Could you check a few things on this model? Use its own coordinates, in mm. A direction names the side the tool comes from. Round coordinates to 2 decimals unless told otherwise and drop trailing zeros. Write each loop counter-clockwise with the first axis right and the second up, starting at its lowest first coordinate (ties: lowest second). Pieces come first, ordered by that corner, then holes. Notation, with made-up numbers: M 8.5,1.5 L 12.5,1.5 A29 ccw 12.5,40.5 Z; hole C 17.25,19.25 d4. An arc over 180 degrees is marked long. One line per item, written item: value. Start each with the question number.
(1) I want a section at D-D on x = 17. Please give me the cut outline in (y, z).
(2) If I drill on L1, parallel to X at y = 7.5, z = 15; L2, parallel to X at y = 1.6, z = 0; L3, parallel to Z at x = 0, y = 6.5, over which ranges is the centre line in solid material (lowest first)?
(3) Which directions (+Z, -Z, +X, -X, +Y, -Y) give clear straight access to the entire face, cutting with the end or side of a thin tool? Please do faces 4 (the face through (4, 3, 1)), 5 (the face through (0, 5, -20)), 6 (the face through (0, 8, -12)).
(4) I want a section at A-A on x = 5. Please give me the cut outline in (y, z), and give its area (3 significant figures).
(5) I want a section at B-B on z = 15. Please give me the cut outline in (x, y), and give its area (3 significant figures).
(6) Thinking about a two-plate mould opening in Z: for faces 1 (the face through (-4, 2, 0)), 2 (the face through (0, 5, 20)), 3 (the face through (0, 11, 17)), which applies, released by +Z, released by -Z, zero draft, split by the parting line, or undercut?
(7) I want a section at C-C on y = 8.5. Please give me the cut outline in (x, z), and give its area (3 significant figures).
(8) I'm going to push flat-ended pins straight in: pin 1 Ø1.2 at (x, z) = (-5, 0.5) entering from +Y; pin 2 Ø12 at (x, z) = (10.5, -2.5) entering from +Y; pin 3 Ø1.8 at (x, z) = (17, -15) entering from +Y. Where does each tip first touch, or does it pass through?
```python
from build123d import *

# Parameters (mm, degrees)
SKETCH1_W               = 50
SKETCH1_H               = 40
BOSS_EXTRUDE1_DEPTH     = 5
SKETCH2_R               = 1
CUT_EXTRUDE1_DEPTH      = 33.403703492
SKETCH3_R               = 2
CUT_EXTRUDE2_DEPTH      = 2
SKETCH5_W               = 50
SKETCH5_H               = 8
BOSS_EXTRUDE2_DEPTH     = 6
CUT_EXTRUDE3_DEPTH      = 33.57299495
CUT_EXTRUDE3_DEPTH_BACK = 33.57299495
SKETCH4_R               = 1


with BuildPart() as part:
    # Sketch1 → Boss-Extrude1 (new body)
    with BuildSketch(Plane(origin=(0, 0, 0), x_dir=(1, 0, 0), z_dir=(0, 1, 0))):
        Rectangle(SKETCH1_W, SKETCH1_H)
    extrude(amount=BOSS_EXTRUDE1_DEPTH)

    # Sketch2 → Cut-Extrude1 (cut, through all)
    with BuildSketch(Plane(origin=(0, 5, 0), x_dir=(1, 0, 0), z_dir=(0, 1, 0))):
        with Locations(Location((-5, 0, 0), (0, 0, 270))):
            Circle(SKETCH2_R)
        with Locations(Location((5, 0, 0), (0, 0, 270))):
            Circle(SKETCH2_R)
    extrude(amount=-CUT_EXTRUDE1_DEPTH, mode=Mode.SUBTRACT)

    # Sketch3 → Cut-Extrude2 (cut)
    with BuildSketch(Plane(origin=(0, 5, 0), x_dir=(1, 0, 0), z_dir=(0, 1, 0))):
        with Locations(Location((-5, 0, 0), (0, 0, 270))):
            Circle(SKETCH3_R)
        with Locations(Location((5, 0, 0), (0, 0, 270))):
            Circle(SKETCH3_R)
    extrude(amount=-CUT_EXTRUDE2_DEPTH, mode=Mode.SUBTRACT)

    # Sketch5 → Boss-Extrude2 (add)
    with BuildSketch(Plane(origin=(0, 5, 0), x_dir=(1, 0, 0), z_dir=(0, 1, 0))):
        with Locations((0, 16)):
            Rectangle(SKETCH5_W, SKETCH5_H)
        with Locations((0, -16)):
            Rectangle(SKETCH5_W, SKETCH5_H)
    extrude(amount=BOSS_EXTRUDE2_DEPTH)

    # Sketch4 → Cut-Extrude3 (cut, two sides: drawn at the far end of the back side and taken through both)
    with BuildSketch(Plane(origin=(0, 5, 0), x_dir=(1, 0, 0), z_dir=(0, 1, 0)).offset(-CUT_EXTRUDE3_DEPTH_BACK)):
        with Locations(Location((-17, 15, 0), (0, 0, 270))):
            Circle(SKETCH4_R)
        with Locations(Location((0, 15, 0), (0, 0, 270))):
            Circle(SKETCH4_R)
        with Locations(Location((17, 15, 0), (0, 0, 270))):
            Circle(SKETCH4_R)
        with Locations(Location((-17, -15, 0), (0, 0, 270))):
            Circle(SKETCH4_R)
        with Locations(Location((0, -15, 0), (0, 0, 270))):
            Circle(SKETCH4_R)
        with Locations(Location((17, -15, 0), (0, 0, 270))):
            Circle(SKETCH4_R)
    extrude(amount=CUT_EXTRUDE3_DEPTH + CUT_EXTRUDE3_DEPTH_BACK, mode=Mode.SUBTRACT)


solid = part.part
```
Found:
1. outline: M 0,-20 L 11,-20 L 11,-16 L 0,-16 Z; M 0,-14 L 11,-14 L 11,-12 L 5,-12 L 5,12 L 11,12 L 11,14 L 0,14 Z; M 0,16 L 11,16 L 11,20 L 0,20 Z
2. L1: x = -25 to -18, -16 to -1, 1 to 16, 18 to 25
2. L2: x = -25 to -6, -4 to 4, 6 to 25
2. L3: z = -20 to -16, -14 to -12, 12 to 14, 16 to 20
3. face 4: +Y
3. face 5: -Z, +X, -X, +Y, -Y
3. face 6: +X, -X, +Y
4. outline: M 0,-20 L 11,-20 L 11,-12 L 5,-12 L 5,-2 L 3,-2 L 3,-1 L 0,-1 Z; M 0,1 L 3,1 L 3,2 L 5,2 L 5,12 L 11,12 L 11,20 L 0,20 Z
4. area: 282 mm²
5. outline: M -25,0 L -18,0 L -18,11 L -25,11 Z; M -16,0 L -1,0 L -1,11 L -16,11 Z; M 1,0 L 16,0 L 16,11 L 1,11 Z; M 18,0 L 25,0 L 25,11 L 18,11 Z
5. area: 484 mm²
6. face 1: undercut
6. face 2: released by +Z
6. face 3: zero draft
7. outline: M -25,-20 L 25,-20 L 25,-12 L -25,-12 Z; M -25,12 L 25,12 L 25,20 L -25,20 Z; hole C -17,-15 d2; hole C -17,15 d2; hole C 0,-15 d2; hole C 0,15 d2; hole C 17,-15 d2; hole C 17,15 d2
7. area: 781 mm²
8. pin 1: stops at y = 3
8. pin 2: stops at y = 5
8. pin 3: passes through
